Part model, mm, in its own coordinate system. Face numbers are marked on the shaded views. A direction names the side the tool comes from. Give positions to 0.01 mm unless a question says otherwise; leave off trailing zeros. Write each loop counter-clockwise with the first axis right and the second up, starting at its lowest first coordinate (ties: lowest second). Pieces come first, ordered by that corner, then holes. Notation, with made-up numbers: M 41,40.5 L 74,40.5 A14 ccw 74,49.5 Z; hole C 84.5,-31.75 d6. An arc over 180 degrees is marked long. Use CSV: the item, a comma, the result in double quotes. Start each with the question number.
Item 1: Drill centre lines: line 1 (Z direction, x = 10, y = -14.4); line 2 (X direction, y = -14.4, z = -21.25); line 3 (Z direction, x = 7, y = 1). Where is each one in solid material? Low to high. Write a range as [from, to].
Item 2: Mould opens along Z. For the marked faces 1, 2 and 3 say: released by +Z, released by -Z, zero draft, split by the parting line, or undercut.
Item 3: Cut at A-A (x = 10). List the corners of the cut face in (y, z), then the cut area to 3 significant figures.
Item 4: Cut at B-B (y = 1.75). List the corners of the cut face in (x, z).
Item 5: Cut at D-D (z = 15). List the corners of the cut face in (x, y), then the cut area to 3 significant figures.
Item 6: Pin check, flat tip, straight feed: pin 1 (10 mm diameter, centred on x = 9.5, z = -13, fed in from +Y). Stop position of the tip, or through.
Item 7: Which spindle directions (+Z, -Z, +X, -X, +Y, -Y) get a long thin tool onto all of the face, cutting with end or side? Do the marked faces 4 and 5. Say none if no direction does.
Item 8: Cut at C-C (z = -21.25). List the corners of the cut face in (x, y), then the cut area to 3 significant figures.
from build123d import *

# Parameters (mm, degrees)
F0_W           = 29
F0_H           = 62.5
F0_W_2         = 25
F0_H_2         = 58.5
F1_DEPTH       = 20
F2_W           = 20
F2_H           = 52.5
F3_DEPTH       = 2
F5_D           = 3.3
F5_CSINK_D     = 6.72
F5_CSINK_ANGLE = 90
F6_DEPTH       = 2
F7_DEPTH       = 2


with BuildPart() as f1:
    # F0 (on Right) → F1 (new body)
    with BuildSketch(Plane.YZ):
        Rectangle(F0_W, F0_H)
        Rectangle(F0_W_2, F0_H_2, mode=Mode.SUBTRACT)
    extrude(amount=F1_DEPTH)

    # F2 (on face) → F3 (cut)
    with BuildSketch(Plane(origin=(0, 14.5, 0), x_dir=(-1, 0, 0), z_dir=(0, 1, 0))):
        with Locations((-10, 0)):
            Rectangle(F2_W, F2_H)
    extrude(amount=-F3_DEPTH, mode=Mode.SUBTRACT)

    # F5 (through all)
    with Locations(Plane(origin=(0, -12.5, 0), x_dir=(-1, 0, 0), z_dir=(0, 1, 0))):
        with Locations((-10, 21.25), (-10, -21.25)):
            CounterSinkHole(F5_D / 2, F5_CSINK_D / 2, counter_sink_angle=F5_CSINK_ANGLE)

    # F6 (add): a face of the model
    f6_faces = [f1.faces().sort_by_distance(p)[0] for p in [
        (10, 13.5, 26.25),
    ]]
    extrude(f6_faces, amount=F6_DEPTH)

    # F7 (add): a face of the model
    f7_faces = [f1.faces().sort_by_distance(p)[0] for p in [
        (10, 13.5, -26.25),
    ]]
    extrude(f7_faces, amount=F7_DEPTH)


solid = f1.part
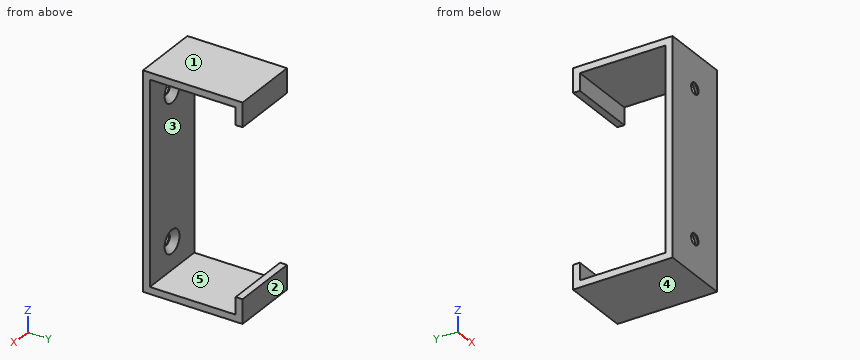
Worked answers:
1,line 1,"z = [-31.25, -22.9], [-19.6, 19.6], [22.9, 31.25]"
1,line 2,"x = [0, 8.35], [11.65, 20]"
1,line 3,"z = [-31.25, -29.25], [29.25, 31.25]"
2,face 1,"released by +Z"
2,face 2,"zero draft"
2,face 3,"undercut"
3,outline,"M -14.5,-31.25 L 14.5,-31.25 L 14.5,-24.25 L 12.5,-24.25 L 12.5,-29.25 L -12.5,-29.25 L -12.5,-24.61 L -14.21,-22.9 L -14.5,-22.9 Z; M -14.5,-19.6 L -14.21,-19.6 L -12.5,-17.89 L -12.5,17.89 L -14.21,19.6 L -14.5,19.6 Z; M -14.5,22.9 L -14.21,22.9 L -12.5,24.61 L -12.5,29.25 L 12.5,29.25 L 12.5,24.25 L 14.5,24.25 L 14.5,31.25 L -14.5,31.25 Z"
3,area,"234 mm^2"
4,outline,"M 0,-31.25 L 20,-31.25 L 20,-29.25 L 0,-29.25 Z; M 0,29.25 L 20,29.25 L 20,31.25 L 0,31.25 Z"
5,outline,"M 0,-14.5 L 20,-14.5 L 20,-12.5 L 0,-12.5 Z"
5,area,"40.0 mm^2"
6,pin 1,"stops at y = -12.5"
7,face 4,"-Z, +X, -X, +Y, -Y"
7,face 5,"+X, -X"
8,outline,"M 0,-14.5 L 8.35,-14.5 L 8.35,-14.21 L 6.64,-12.5 L 0,-12.5 Z; M 11.65,-14.5 L 20,-14.5 L 20,-12.5 L 13.36,-12.5 L 11.65,-14.21 Z"
8,area,"30.5 mm^2"
